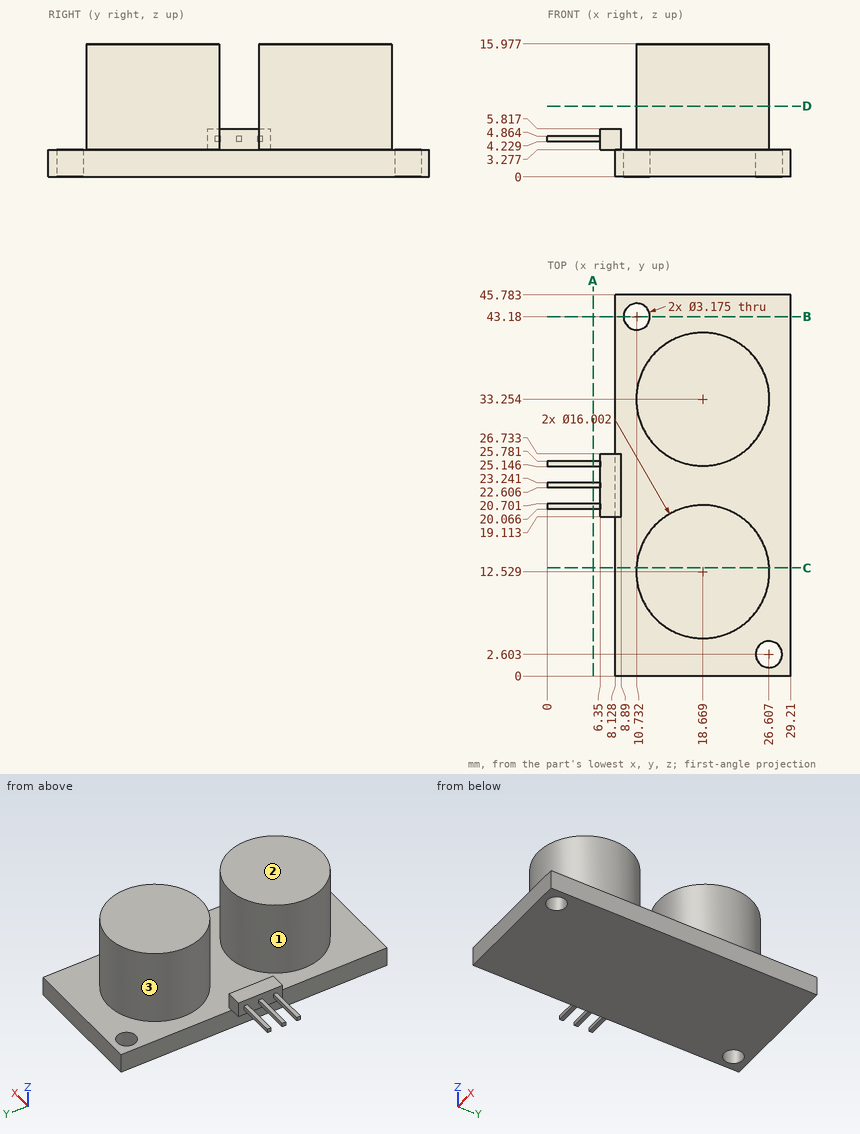
Check sheet for the drawn part. Datum: minimum x, y, z corner. Units: mm. Round coordinates to 2 decimals unless told otherwise and drop trailing zeros. Write each loop counter-clockwise with the first axis right and the second up, starting at its lowest first coordinate (ties: lowest second). Pieces come first, ordered by that corner, then holes. Notation, with made-up numbers: (-1, 5) - (35, 5) arc R21 cw to (35, 21) - close; hole circle Ø9 at (-25, 22.5). An arc over 180 degrees is marked (long way). Write each question's results on one line, items separated by ' | '.
(1) Sectioned sample at B-B, the plane y = 43.18. Enter the section's corners in (x, z) (1 decimal).
Computed:
outline: (8.1, 0) - (9.1, 0) - (9.1, 3.3) - (8.1, 3.3) - close; (12.3, 0) - (29.2, 0) - (29.2, 3.3) - (12.3, 3.3) - close
(2) Depth check by flat-ended pin: pin 1 Ø3 at (x, z) = (7, 5) entering from +Y; pin 2 Ø2.5 at (y, z) = (15.5, 2.5) entering from -X; pin 3 Ø8 at (y, z) = (25.5, 11) entering from +X (1 decimal); pin 4 Ø3 at (x, y) = (26.61, 2.6) entering from -Z. Enter the tip coordinate at first touch or a pass-through.
Computed:
pin 1: stops at y = 26.73 | pin 2: stops at x = 8.13 | pin 3: stops at x = 25.7 | pin 4: passes through
(3) Draft check along Y on the marked faces 1, 2 and 3. Enter one of: pulls with the +Y half, pulls with the -Y half, needs draft (parallel to the pull), parting line crosses it, or undercut.
Computed:
face 1: undercut | face 2: needs draft | face 3: undercut
(4) Thickness scan on probe 1 along Y at (x, z) = (2.5, 4.75) (1 decimal); probe 2 along X at (y, z) = (43.18, 2.25) (1 decimal); probe 3 along X at (y, z) = (10.5, 2.5). Record the ranges inside material, lowest first. Write a range as from..to.
Computed:
probe 1: y = 20.1..20.7, 22.6..23.2, 25.1..25.8 | probe 2: x = 8.1..9.1, 12.3..29.2 | probe 3: x = 8.13..29.21
(5) Sectioned sample at C-C, the plane y = 13. Enter the section's corners in (x, z), plus the area to 3 significant figures.
Computed:
outline: (8.13, 0) - (29.21, 0) - (29.21, 3.28) - (26.66, 3.28) - (26.66, 15.98) - (10.68, 15.98) - (10.68, 3.28) - (8.13, 3.28) - close | area: 272 mm^2
(6) Sectioned sample at A-A, the plane x = 5.5. Enter the section's corners in (y, z) (1 decimal).
Computed:
outline: (20.1, 4.2) - (20.7, 4.2) - (20.7, 4.9) - (20.1, 4.9) - close; (22.6, 4.2) - (23.2, 4.2) - (23.2, 4.9) - (22.6, 4.9) - close; (25.1, 4.2) - (25.8, 4.2) - (25.8, 4.9) - (25.1, 4.9) - close
(7) Sectioned sample at D-D, the plane z = 8.5. Enter the section's corners in (x, y) (1 decimal), plus the area to 3 significant figures.
Computed:
outline: circle Ø16 at (18.7, 12.5); circle Ø16 at (18.7, 33.3) | area: 402 mm^2
